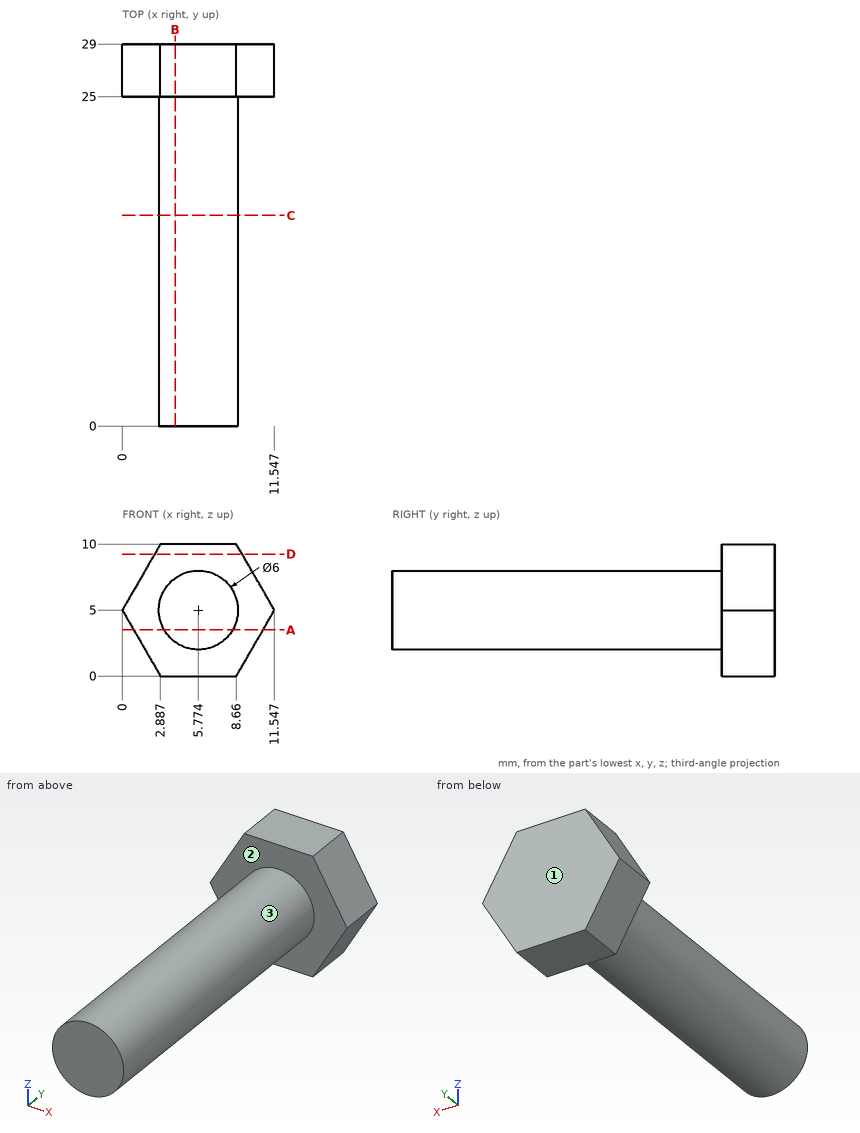
Answer from the drawing. Dimensions are ordinates in mm from the lowest x, y and z of the part. Give positions to 0.01 mm unless a question says otherwise; leave off trailing zeros. Loops run counter-clockwise (first coordinate to the right, second up) from the corner with the lowest first, then second, coordinate; pieces in that order, holes last. Notation, with made-up numbers: (2.5, 50) - (35.5, 50) arc R13 cw to (35.5, 70) - close; hole circle Ø4 at (89.5, 66.5). An arc over 180 degrees is marked (long way). Answer as a JSON object with one key per item and string values.
1. For a pull along Y with two mould halves and no side action, classify the marked faces 1, 2 and 3 as pulls with the +Y half, pulls with the -Y half, needs draft (parallel to the pull), parting line crosses it, or undercut.
Determined:
{"face 1": "pulls with the +Y half", "face 2": "pulls with the -Y half", "face 3": "needs draft"}
2. A cutting plane is placed at B-B (x = 4). Write down the section's boundary in (y, z), then the cut area to 3 significant figures.
Determined:
{"outline": "(0, 2.58) - (25, 2.58) - (25, 0) - (29, 0) - (29, 10) - (25, 10) - (25, 7.42) - (0, 7.42) - close", "area": "161 mm²"}
3. Flat-ended cylindrical pins translate along their axes: pin 1 Ø4 at (x, y) = (2, 19.5) entering from +Z; pin 2 Ø3 at (y, z) = (20, 3) entering from +X; pin 3 Ø3 at (x, z) = (1.5, 7.5) entering from -Y. Find the tip coordinate at first contact, or state that the pin passes through.
Determined:
{"pin 1": "z = 7.42", "pin 2": "x = 8.73", "pin 3": "y = 25"}
4. A cutting plane is placed at D-D (z = 9.25). Write down the section's boundary in (x, y).
Determined:
{"outline": "(2.45, 25) - (9.09, 25) - (9.09, 29) - (2.45, 29) - close"}
5. Find the intervals of material crossed by L1, parallel to Y at x = 2.5, z = 9.25; L2, parallel to X at y = 16.25, z = 7.25 (1 decimal); L3, parallel to Z at x = 5.25, y = 22.75 (1 decimal), in increasing order. Write a range as [from, to].
Determined:
{"L1": "[25, 29]", "L2": "[3.8, 7.8]", "L3": "[2, 8]"}
6. A cutting plane is placed at A-A (z = 3.5). Write down the section's boundary in (x, y) (1 decimal).
Determined:
{"outline": "(0.9, 25) - (3.2, 25) - (3.2, 0) - (8.4, 0) - (8.4, 25) - (10.7, 25) - (10.7, 29) - (0.9, 29) - close"}
7. A cutting plane is placed at C-C (y = 16). Write down the section's boundary in (x, z), then the cut area to 3 significant figures.
Determined:
{"outline": "circle Ø6 at (5.77, 5)", "area": "28.3 mm²"}
